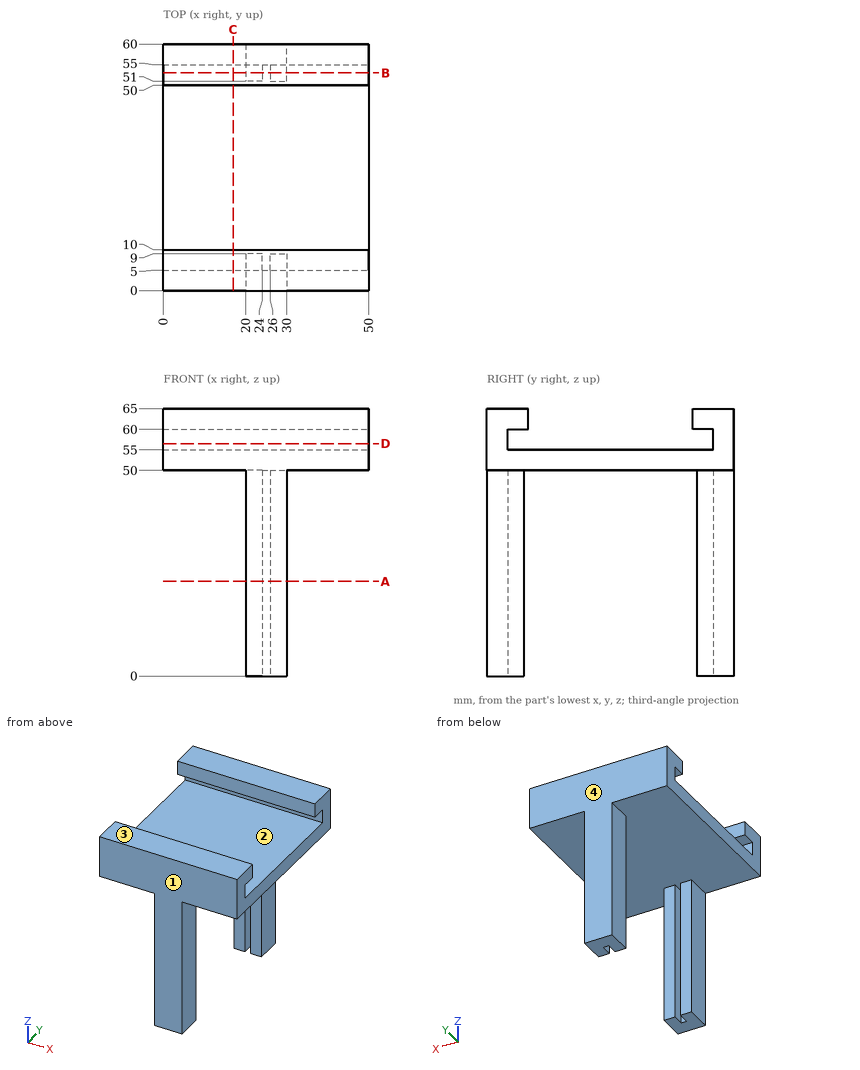
Here's the drawing with two shaded views (mm, measured from the low corner). I have some questions. Give positions to 0.01 mm unless a question says otherwise; leave off trailing zeros. Write each loop counter-clockwise with the first axis right and the second up, starting at its lowest first coordinate (ties: lowest second). Pieces come first, ordered by that corner, then holes. Notation, with made-up numbers: (53.5, 3.5) -> (112.5, 3.5) arc R33 cw to (112.5, 42.5) -> close; hole circle Ø11 at (28.25, 71.25). An arc over 180 degrees is marked (long way). Answer as a JSON object with one key per item and string values. Group by question number.
Item 1: We'd pull the mould along Y, two halves only. Please class the marked faces 1, 2, 3 and 4: +Y half, -Y half, draft (parallel to the pull), parting line (faces both ways), or undercut.
Item 2: Suppose I cut it at C-C (x = 17). Please give me the cut outline in (y, z), plus the area to 3 significant figures.
Item 3: Suppose I cut it at B-B (y = 53). Please give me the cut outline in (x, z).
Item 4: Suppose I cut it at A-A (z = 23). Please give me the cut outline in (x, y), plus the area to 3 significant figures.
Item 5: I'm going to push flat-ended pins straight in: P1, Ø1.5, axis at x = 38.5, y = 20, coming from the -Z side; P2, Ø3, axis at y = 52, z = 23, coming from the -X side; P3, Ø4.5, axis at y = 53.5, z = 33, coming from the +X side; P4, Ø10, axis at y = 15.5, z = 19.5, coming from the +X side. Where does each tip first touch, or does it pass through?
Item 6: Please list where these lines run through material, in increasing order: line 1 (Y direction, x = 23, z = 11); line 2 (Z direction, x = 44, y = 9.5); line 3 (Z direction, x = 8.5, y = 17). Write a range as [from, to].
Item 7: Suppose I cut it at D-D (z = 56.5). Please give me the cut outline in (x, y).
Findings:
{
 "1": {"face 1": "-Y half", "face 2": "undercut", "face 3": "draft", "face 4": "+Y half"},
 "2": {"outline": "(0, 50) -> (60, 50) -> (60, 65) -> (50, 65) -> (50, 60) -> (55, 60) -> (55, 55) -> (5, 55) -> (5, 60) -> (10, 60) -> (10, 65) -> (0, 65) -> close", "area": "450 mm²"},
 "3": {"outline": "(0, 50) -> (20, 50) -> (20, 0) -> (24, 0) -> (24, 50) -> (26, 50) -> (26, 0) -> (30, 0) -> (30, 50) -> (50, 50) -> (50, 55) -> (0, 55) -> close; (0, 60) -> (50, 60) -> (50, 65) -> (0, 65) -> close"},
 "4": {"outline": "(20, 0) -> (30, 0) -> (30, 9) -> (26, 9) -> (26, 5) -> (24, 5) -> (24, 9) -> (20, 9) -> close; (20, 51) -> (24, 51) -> (24, 55) -> (26, 55) -> (26, 51) -> (30, 51) -> (30, 60) -> (20, 60) -> close", "area": "164 mm²"},
 "5": {"P1": "stops at z = 50", "P2": "stops at x = 20", "P3": "stops at x = 30", "P4": "passes through"},
 "6": {"line 1": "y = [0, 9], [51, 60]", "line 2": "z = [50, 55], [60, 65]", "line 3": "z = [50, 55]"},
 "7": {"outline": "(0, 0) -> (50, 0) -> (50, 5) -> (0, 5) -> close; (0, 55) -> (50, 55) -> (50, 60) -> (0, 60) -> close"}
}
